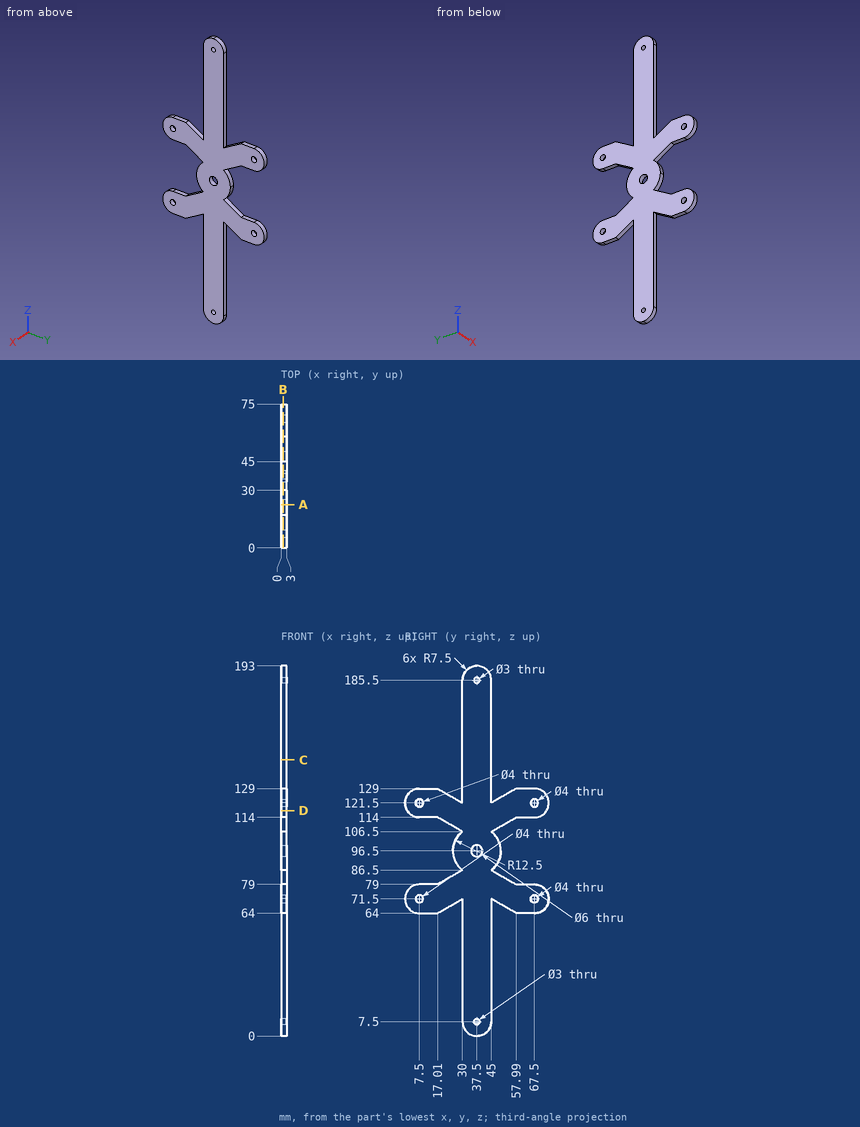
Input: dimensioned drawing with shaded views. Units: mm. Origin: part minimum x, y, z. Round coordinates to 2 decimals unless told otherwise and drop trailing zeros. Order: outer loops, then holes, each group sorted by start corner. A loop starts at its lowest first (then second) coordinate and runs counter-clockwise, first axis right, second up. Notation, with made-up numbers: (87.5, 75) - (132.5, 75) arc R21 ccw to (132.5, 94) - close; hole circle Ø1 at (52.5, 30.25). An arc over 180 degrees is marked (long way). Write item = value, one per line. Start each with the question number.
Q1. Pin query (flat end, axial travel): pin 1 (1.5 mm diameter, centred on x = 2.5, y = 9.5, fed in from +Z); pin 2 (0.9 mm diameter, centred on x = 1.5, z = 27.5, fed in from +Y); pin 3 (4 mm diameter, centred on y = 34, z = 20, fed in from -X); pin 4 (1.5 mm diameter, centred on x = 1.5, y = 64.5, fed in from -Z). Return the tip coordinate at first contact, or that it passes through.
Q2. Cut plane A-A on y = 22.5. Return the cut outline in (x, z).
Q3. Cut plane C-C on z = 144. Return the cut outline in (x, y), and give its area (3 significant figures).
Q4. Ray query, line 1 (Z direction, x = 1.9, y = 7.5); line 2 (Z direction, x = 2.15, y = 16); line 3 (Y direction, x = 1.2, z = 65) (1 decimal). Return the intervals inside material, ascending. Write a range as from..to.
Q5. Cut plane D-D on z = 117.5. Return the cut outline in (x, y) (1 decimal).
Q6. Cut plane B-B on x = 0.95. Give the number of separate pieces and of enclosed holes in the cut face, and give its area (3 significant figures).
Outcome:
q1.pin_1 = 129
q1.pin_2 = 45
q1.pin_3 = 0
q1.pin_4 = 64
q2.outline = (0, 67.17) - (3, 67.17) - (3, 82.17) - (0, 82.17) - close; (0, 110.83) - (3, 110.83) - (3, 125.83) - (0, 125.83) - close
q3.outline = (0, 30) - (3, 30) - (3, 45) - (0, 45) - close
q3.area = 45.0 mm^2
q4.line_1 = 64..69.5, 73.5..79, 114..119.5, 123.5..129
q4.line_2 = 64..79, 114..129
q4.line_3 = 3.8..18.7, 30..45, 56.3..71.2
q5.outline = (0, 1.2) - (3, 1.2) - (3, 73.8) - (0, 73.8) - close
q6.separate_pieces = 1
q6.enclosed_holes = 7
q6.area = 4,600 mm^2
